Could you check a few things on this model? Use its own coordinates, in mm. Face numbers are marked on the shaded views. A direction names the side the tool comes from. Give positions to 0.01 mm unless a question says otherwise; leave off trailing zeros. Write each loop counter-clockwise with the first axis right and the second up, starting at its lowest first coordinate (ties: lowest second). Pieces come first, ordered by that corner, then holes. Notation, with made-up numbers: M 27.25,-3.75 L 65.25,-3.75 A31 cw 65.25,35.25 Z; hole C 27.5,51.5 d6. An arc over 180 degrees is marked long. Use one line per item in the form item = value.
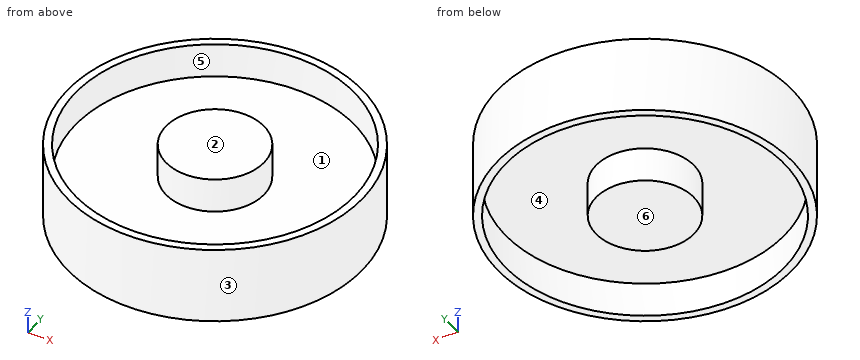
from build123d import *

# Parameters (mm, degrees)
SKETCH1_R           = 18.05
SKETCH1_R_2         = 6.35
BOSS_EXTRUDE1_DEPTH = 0.5
SKETCH1_3_R         = 19.05
SKETCH1_3_R_2       = 18.05
SKETCH1_3_R_3       = 6.35
BOSS_EXTRUDE2_DEPTH = 5


with BuildPart() as part:
    # Sketch1 → Boss-Extrude1 (new, symmetric)
    with BuildSketch(Plane.XY):
        Circle(SKETCH1_R)
        Circle(SKETCH1_R_2, mode=Mode.SUBTRACT)
    extrude(amount=BOSS_EXTRUDE1_DEPTH, both=True)

    # Sketch1<3> → Boss-Extrude2 (add, symmetric)
    # profile 1 of 2: a face of its own
    with BuildSketch(Plane.XY):
        Circle(SKETCH1_3_R)
        Circle(SKETCH1_3_R_2, mode=Mode.SUBTRACT)
    # profile 2 of 2: a face of its own
    with BuildSketch(Plane.XY):
        Circle(SKETCH1_3_R_3)
    extrude(amount=BOSS_EXTRUDE2_DEPTH, both=True)


solid = part.part
1) I want a section at D-D, the plane x = 16.5. Please give me the cut outline in (y, z).
Checked values:
outline = M -9.52,-5 L -7.32,-5 L -7.32,-0.5 L 7.32,-0.5 L 7.32,-5 L 9.52,-5 L 9.52,5 L 7.32,5 L 7.32,0.5 L -7.32,0.5 L -7.32,5 L -9.52,5 Z
2) For pin 1 Ø1.5 at (x, z) = (11, -3.5) entering from +Y; pin 2 Ø1 at (x, y) = (11, 12) entering from +Z, each with a flat end and sliding along its axis, tell me the tip position at first contact or that it passes through.
Checked values:
pin_1 = 16.06
pin_2 = 0.5
3) If I drill on L1, parallel to Y at x = 0, z = -3.35; L2, parallel to X at y = 3.5, z = 3.25; L3, parallel to Z at x = 1.5, y = 14, over which ranges is the centre line in solid material (lowest first)?
Checked values:
L1 = -19.05 to -18.05, -6.35 to 6.35, 18.05 to 19.05
L2 = -18.73 to -17.71, -5.3 to 5.3, 17.71 to 18.73
L3 = -0.5 to 0.5
4) For the marked faces 4, 5 and 6, which set-ups out of +Z, -Z, +X, -X, +Y, -Y let a thin tool reach every point of the face, with its end or its side?
Checked values:
face_4 = -Z
face_5 = +Z
face_6 = -Z, +X, -X, +Y, -Y
5) I want a section at B-B, the plane x = 0. Please give me the cut outline in (y, z), plus the area to 3 significant figures.
Checked values:
outline = M -19.05,-5 L -18.05,-5 L -18.05,-0.5 L -6.35,-0.5 L -6.35,-5 L 6.35,-5 L 6.35,-0.5 L 18.05,-0.5 L 18.05,-5 L 19.05,-5 L 19.05,5 L 18.05,5 L 18.05,0.5 L 6.35,0.5 L 6.35,5 L -6.35,5 L -6.35,0.5 L -18.05,0.5 L -18.05,5 L -19.05,5 Z
area = 170 mm2
6) Thinking about a two-plate mould opening in X: for the marked faces 1, 2 and 3, which applies, released by +X, released by -X, zero draft, split by the parting line, or undercut?
Checked values:
face_1 = undercut
face_2 = zero draft
face_3 = split by the parting line
7) I want a section at A-A, the plane z = 2.75. Please give me the cut outline in (x, y), plus the area to 3 significant figures.
Checked values:
outline = C 0,0 d38.1; C 0,0 d12.7; hole C 0,0 d36.1
area = 243 mm2
